Can you work these out from the model? Positions are in its coordinate system, mm. Face numbers are marked on the shaded views. A direction names the side the tool comes from. Round coordinates to 2 decimals unless told otherwise and drop trailing zeros. Loops run counter-clockwise (first coordinate to the right, second up) from the corner with the lowest first, then second, coordinate; pieces in that order, holes last.
```python
from build123d import *

# Parameters (mm, degrees)
F1_DEPTH = 8.5


with BuildPart() as f1:
    # F0 (on Top) → F1 (new body)
    with BuildSketch(Plane.XY):
        Polygon((-4, 2.1), (-4, 0), (-2, 0), (-2, 2.1), (3, 2.1), (3, 5.1), (-5, 5.1), (-7, 5.1), (-9, 5.1), (-11, 5.1), (-13, 5.1), (-15, 5.1), (-17, 5.1), (-19, 5.1), (-21, 5.1), (-32, 5.1), (-32, 2.1), (-32, 1.1), (-30, 1.1), (-30, 2.1), (-28, 2.1), (-28, 1.1), (-26, 1.1), (-26, 2.1), align=None)
        Polygon((-2, 0), (-4, 0), (-4, -2.1), (-26, -2.1), (-26, -1.1), (-28, -1.1), (-28, -2.1), (-30, -2.1), (-30, -1.1), (-32, -1.1), (-32, -2.1), (-32, -5.1), (-21, -5.1), (-19, -5.1), (-17, -5.1), (-15, -5.1), (-13, -5.1), (-11, -5.1), (-9, -5.1), (-7, -5.1), (-5, -5.1), (3, -5.1), (3, -2.1), (-2, -2.1), align=None)
        Polygon((-7, 5.1), (-5, 5.1), (-6, 6.1), align=None)
        Polygon((-6, -6.1), (-5, -5.1), (-7, -5.1), align=None)
        Polygon((-9, 5.1), (-7, 5.1), (-8, 6.1), align=None)
        Polygon((-8, -6.1), (-7, -5.1), (-9, -5.1), align=None)
        Polygon((-11, 5.1), (-9, 5.1), (-10, 6.1), align=None)
        Polygon((-10, -6.1), (-9, -5.1), (-11, -5.1), align=None)
        Polygon((-13, 5.1), (-11, 5.1), (-12, 6.1), align=None)
        Polygon((-12, -6.1), (-11, -5.1), (-13, -5.1), align=None)
        Polygon((-15, 5.1), (-13, 5.1), (-14, 6.1), align=None)
        Polygon((-14, -6.1), (-13, -5.1), (-15, -5.1), align=None)
        Polygon((-17, 5.1), (-15, 5.1), (-16, 6.1), align=None)
        Polygon((-16, -6.1), (-15, -5.1), (-17, -5.1), align=None)
        Polygon((-19, 5.1), (-17, 5.1), (-18, 6.1), align=None)
        Polygon((-18, -6.1), (-17, -5.1), (-19, -5.1), align=None)
        Polygon((-20, 6.1), (-21, 5.1), (-19, 5.1), align=None)
        Polygon((-19, -5.1), (-21, -5.1), (-20, -6.1), align=None)
    extrude(amount=F1_DEPTH)


solid = f1.part
```
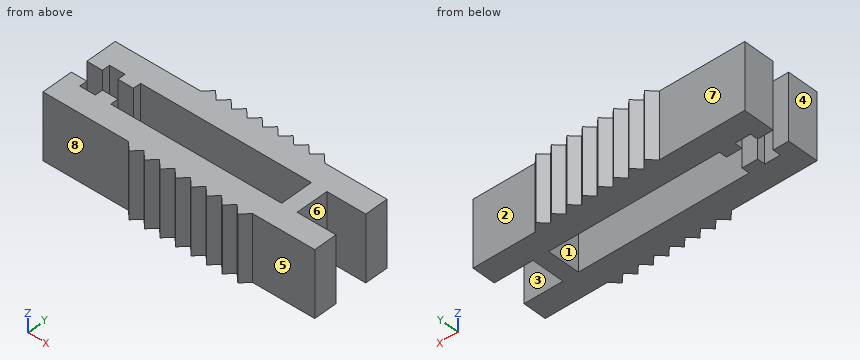
(1) For pin 1 (0.6 mm diameter, centred on x = -27.5, z = 6.5, fed in from +Y); pin 2 (1 mm diameter, centred on x = -31, z = 6, fed in from -Y); pin 3 (1.1 mm diameter, centred on y = -1.5, z = 4.5, fed in from +X), each with a flat end and sliding along its axis, tell me the tip position at first contact or that it passes through.
(2) Which directions (+Z, -Z, +X, -X, +Y, -Y) give clear straight access to the entire face, cutting with the end or side of a thin tool? Please do the marked faces 1, 2, 3, 4 and 5.
(3) Suppose I cut it at C-C (x = -0.5). Write out the boundary of the cut face in (y, z), then the cut area to 3 significant figures.
(4) Suppose I cut it at B-B (y = 1.75). Write out the boundary of the cut face in (x, z).
(5) Suppose I cut it at D-D (y = -0.25). Write out the boundary of the cut face in (x, z), then the cut area to 3 significant figures.
(6) If I drill on line 1 (X direction, y = 1.25, z = 6); line 2 (Y direction, x = 0, z = 6); line 3 (X direction, y = -1, z = 4.25), over which ranges is the centre line in solid material (lowest first)?
(7) Suppose I cut it at A-A (x = -18.5). Write out the boundary of the cut face in (y, z).
(8) We'd pull the mould along Y, two halves only. Please class the marked faces 6, 7 and 8: released by +Y, released by -Y, zero draft, split by the parting line, or undercut.
Check result:
1. pin 1: stops at y = 5.1
1. pin 2: stops at y = -5.1
1. pin 3: stops at x = -2
2. face 1: +Z, -Z
2. face 2: +Z, -Z, +X, +Y
2. face 3: +Z, -Z, +X
2. face 4: +Z, -Z, -X, +Y, -Y
2. face 5: +Z, -Z, +X, -Y
3. outline: (-5.1, 0) - (-2.1, 0) - (-2.1, 8.5) - (-5.1, 8.5) - close; (2.1, 0) - (5.1, 0) - (5.1, 8.5) - (2.1, 8.5) - close
3. area: 51.0 mm2
4. outline: (-32, 0) - (-30, 0) - (-30, 8.5) - (-32, 8.5) - close; (-28, 0) - (-26, 0) - (-26, 8.5) - (-28, 8.5) - close; (-4, 0) - (-2, 0) - (-2, 8.5) - (-4, 8.5) - close
5. outline: (-4, 0) - (-2, 0) - (-2, 8.5) - (-4, 8.5) - close
5. area: 17.0 mm2
6. line 1: x = -32 to -30, -28 to -26, -4 to -2
6. line 2: y = -5.1 to -2.1, 2.1 to 5.1
6. line 3: x = -4 to -2
7. outline: (-5.6, 0) - (-2.1, 0) - (-2.1, 8.5) - (-5.6, 8.5) - close; (2.1, 0) - (5.6, 0) - (5.6, 8.5) - (2.1, 8.5) - close
8. face 6: undercut
8. face 7: released by +Y
8. face 8: released by -Y
